Autodesk Inventor part; units mm, degrees
ref_plane "YZ Plane" through (0, 0, 0) normal (1, 0, 0) x (0, 1, 0)
ref_plane "XZ Plane" through (0, 0, 0) normal (0, 1, 0) x (-1, 0, 0)
ref_plane "XY Plane" through (0, 0, 0) normal (0, 0, 1) x (1, 0, 0)
sketch "Sketch1" plane through (0, 0, 0) normal (0, 0, 1) x (1, 0, 0)
  circle A0 centre (0, 0) radius 350
  circle A1 centre (0, 0) radius 380
  line L0 (0, 0) -> (-268.7006, 268.7006)
  line L1 (0, 0) -> (0, 380)
  line L2 (0, 0) -> (268.7006, 268.7006)
  point P0 (-247.4874, 247.4874)
  point P1 (247.4874, 247.4874)
  dimension "d30" = 90
  dimension "d31" = 760
  dimension "d32" = 700
extrude "Plate1" add sketch "Sketch1" against normal blind 2 contours A0 L1 A1 L2 | L0 A1 L1 A0
sketch "Sketch2" plane through (0, 0, 0) normal (0, 0, 1) x (1, 0, 0)
  circle A0 centre (0, 0) radius 367.5
  arc A1 (268.7006, 268.7006) -> (-268.7006, 268.7006) centre (0, 0) ccw
  line L0 (0, 0) -> (268.7006, 268.7006) construction
  line L1 (0, 0) -> (246.7979, 272.2995) construction
  line L2 (157.1265, 332.2161) -> (0, 0) construction
  line L3 (0, 0) -> (0, 367.5) construction
  line L4 (0, 0) -> (18.0324, 367.0573) construction
  line L5 (0, 0) -> (123.807, 346.0174) construction
  dimension "d34" = 735
  dimension "d35" = 2.812
  dimension "d36" = 16.875
  dimension "d44" = 2.812
  dimension "d45" = 16.875
hole "Hole1" at (246.7979, 272.2995, 0) at (157.1265, 332.2161, 0) at (123.807, 346.0174, 0) at (18.0324, 367.0573, 0) direction (0, 0, -1) diameter 8 end through all
pattern_circular "Circular Pattern1" count 2 over 45 about axis through (0, 0, -10) along (0, 0, 1) of "Hole1"
equation "\"d31\" = Колесо_диам_1"
equation "\"d32\" = Колесо_диам_2"
equation "\"d44\" = d35"
equation "\"d45\" = d36"
equation "\"d42\" = Thickness"
equation "\"d15\" = Thickness"
equation "\"BendRadius\" = Thickness"
equation "\"BendReliefWidth\" = Thickness"
equation "\"BendReliefDepth\" = 0.5 * Thickness"
equation "\"CornerReliefSize\" = 4 * Thickness"
equation "\"MinimumRemnant\" = 2 * Thickness"
equation "\"TransitionRadius\" = BendRadius"
equation "\"JacobiRadiusSize\" = BendRadius"
equation "\"GapSize\" = Thickness"
properties part number "DMF2.0 01 43 Gear rim 3"
The listing builds one solid part. Answer for the finished solid, in the listing's coordinates (mm). Round coordinates to 2 decimals unless told otherwise and drop trailing zeros. Write each loop counter-clockwise with the first axis right and the second up, starting at its lowest first coordinate (ties: lowest second). Pieces come first, ordered by that corner, then holes. Notation, with made-up numbers: (54.25, 76.5) -> (66.25, 76.5) arc R24 cw to (66.25, 104.5) -> close; hole circle Ø3 at (78.5, -2.5). An arc over 180 degrees is marked (long way). Answer as a JSON object with one key per item and string values. Group by question number.
Q1. Section D-D (x = -94) is taken. Write down the section's boundary in (y, z).
Q2. Section C-C (x = -30) is taken. Write down the section's boundary in (y, z).
Q3. Determine the mould class of faces 1 (the face through (4.178, 379.977, -0.986)), 2 (the face through (-1, 358, -2)), 3 (the face through (3.85, 349.98, -0.99)) for opening direction X: pulls with the +X half, pulls with the -X half, needs draft (parallel to the pull), parting line crosses it, or undercut.
Q4. Section A-A (y = 303.5) is taken. Write down the section's boundary in (x, z), plus the area to 3 significant figures.
Q5. This flat-tipped pin is pushed along its axis until it touches: pin 1 Ø1 at (y, z) = (328, -1) entering from +X. Where does it stop, or does it pass through?
Q6. Straight lines are drawn through the part: line 1 along X through (y, z) = (301.5, -1.6); line 2 along X through (y, z) = (306, -0.75); line 3 along Y through (x, z) = (18.5, -1.55). For each, find the intervals that lie inside material, in ascending order.
Check values:
{
 "1": {"outline": "(337.14, -2) -> (368.19, -2) -> (368.19, 0) -> (337.14, 0) -> close"},
 "2": {"outline": "(348.71, -2) -> (378.81, -2) -> (378.81, 0) -> (348.71, 0) -> close"},
 "3": {"face 1": "parting line crosses it", "face 2": "needs draft", "face 3": "undercut"},
 "4": {"outline": "(-228.67, -2) -> (-174.32, -2) -> (-174.32, 0) -> (-228.67, 0) -> close; (174.32, -2) -> (228.67, -2) -> (228.67, 0) -> (174.32, 0) -> close", "area": "217 mm^2"},
 "5": {"pin 1": "x = 192.73"},
 "6": {"line 1": "-231.3 to -177.76, 177.76 to 231.3", "line 2": "-225.31 to -169.89, 169.89 to 225.31", "line 3": "349.51 to 363.08, 371.03 to 379.55"}
}
